Input: part model. Units: mm. Frame: model coordinates. A direction names the side the tool comes from. Coordinates: 2 decimals unless noted, no trailing zeros. Order: outer loops, then holes, each group sorted by start corner. A loop starts at its lowest first (then second) coordinate and runs counter-clockwise, first axis right, second up.
from build123d import *

# Parameters (mm, degrees)
F0_W       = 76.1181116104
F0_H       = 56.3871376216
F1_DEPTH   = 67.818
F2_W       = 17.9207939655
F2_H       = 17.2872282565
F3_DEPTH   = 66.802
F4_T       = -2.54
F5_W       = 17.5273697823
F5_H       = 13.1161464378
F1_FACE2_W = 76.1181116104
F1_FACE2_H = 56.3871376216
F6_DEPTH   = 0.508


with BuildPart() as f1:
    # F0 (on Right) → F1 (new body)
    with BuildSketch(Plane.YZ):
        with Locations((38.0590558052, 28.1935688108)):
            Rectangle(F0_W, F0_H)
    extrude(amount=F1_DEPTH)

    # F2 (on face) → F3 (join)
    with BuildSketch(Plane.XZ):
        with Locations((33.3073316142, 8.6436141282)):
            Rectangle(F2_W, F2_H)
    extrude(amount=-F3_DEPTH)

    # F4
    f4_openings = [f1.faces().sort_by_distance(p)[0] for p in [
        (33.909, 38.059056, 0),
    ]]
    offset(amount=F4_T, openings=f4_openings)

    # F5 (on face) + F1_face2 (on face) → F6 (join)
    with BuildSketch(Plane.YZ.offset(67.818)):
        with Locations((35.2515848354, 6.5580732189)):
            Rectangle(F5_W, F5_H)
    with BuildSketch(Plane(origin=(0, 38.0590558052, 28.1935688108), x_dir=(0, 1, 0), z_dir=(-1, 0, 0))):
        Rectangle(F1_FACE2_W, F1_FACE2_H)
    extrude(amount=-F6_DEPTH, dir=(1, 0, 0))


solid = f1.part
Item 1: Cut plane A-A on z = 31. Return loops of the section in (x, y), then the cut area to 3 significant figures.
Response values:
outline: (-0.51, 0) - (67.82, 0) - (67.82, 76.12) - (-0.51, 76.12) - close; hole (2.54, 2.54) - (65.28, 2.54) - (65.28, 73.58) - (2.54, 73.58) - close
area: 744 mm2
Item 2: Cut plane B-B on y = 27.5. Return loops of the section in (x, z), then the cut area to 3 significant figures.
Response values:
outline: (-0.51, 0) - (2.54, 0) - (2.54, 53.85) - (65.28, 53.85) - (65.28, 0) - (67.82, 0) - (67.82, 56.39) - (-0.51, 56.39) - close
area: 474 mm2
Item 3: Pin query (flat end, axial travel): pin 1 Ø5 at (x, y) = (27.5, 8.5) entering from -Z. Return the tip coordinate at first contact, or that it passes through.
Response values:
pin 1: stops at z = 53.85
Item 4: Draft query along Y for faces 3 (the face through (33, 38, 53.847)), 4 (the face through (1, 35, 0)), 5 (the face through (34, 0, 29)), 6 (the face through (34, 76.118, 29)). Return one class per face: pulls with the +Y half, pulls with the -Y half, needs draft (parallel to the pull), parting line crosses it, or undercut.
Response values:
face 3: undercut
face 4: needs draft
face 5: pulls with the -Y half
face 6: pulls with the +Y half
Item 5: Ray query, probe 1 along Y at (x, z) = (42, 31); probe 2 along X at (y, z) = (46, 42.5); probe 3 along Z at (x, y) = (18.5, 52.5). Return the intervals inside material, ascending.
Response values:
probe 1: y = 0 to 2.54, 73.58 to 76.12
probe 2: x = -0.51 to 2.54, 65.28 to 67.82
probe 3: z = 53.85 to 56.39
Item 6: Access query for faces 1 (the face through (33, 73.578, 27)), 2 (the face through (67.818, 38, 29)). Directions: +Z, -Z, +X, -X, +Y, -Y. A direction counts if a zero-diameter tool reaches every point of the face in a straight line with its end or side. Return the directions, or none.
Response values:
face 1: -Z
face 2: +Z, -Z, +X, +Y, -Y
Item 7: Cut plane C-C on x = 53. Return loops of the section in (y, z).
Response values:
outline: (0, 0) - (2.54, 0) - (2.54, 53.85) - (73.58, 53.85) - (73.58, 0) - (76.12, 0) - (76.12, 56.39) - (0, 56.39) - close
